```python
from build123d import *

# Parameters (mm, degrees)
ZAOBLIT1_R = 20


with BuildPart() as part:
    # Skica1 → Rotovat1 (revolve)
    with BuildSketch(Plane.XY, mode=Mode.PRIVATE) as rotovat1_sk:
        Polygon((0, 0), (0, 44.5), (349.599506462, 44.5), (372.134762873, 17.400641026), (420, 17.400641026), (420, 0), align=None)
    revolve(rotovat1_sk.sketch.rotate(Axis((0, 0, 0), (1, 0, 0)), 90), axis=Axis((0, 0, 0), (1, 0, 0)))

    # Zaoblit1
    zaoblit1_edges = [part.edges().sort_by_distance(p)[0] for p in [
        (372.134762873, 0, -17.400641026),
        (349.599506462, 0, -44.5),
        (0, 0, -44.5),
    ]]
    fillet(zaoblit1_edges, radius=ZAOBLIT1_R)


solid = part.part
```
Geometry check sheet. Reference: the model listing, model coordinates, mm. A direction names the side the tool comes from. Give positions to 0.01 mm unless a question says otherwise; leave off trailing zeros. Loops run counter-clockwise (first coordinate to the right, second up) from the corner with the lowest first, then second, coordinate; pieces in that order, holes last. Notation, with made-up numbers: M 42.5,74.5 L 62.5,74.5 A19 ccw 62.5,90.5 Z; hole C 25.25,87 d1. An arc over 180 degrees is marked long. Answer as CSV lines item,"result".
Item 1: Material ranges on line 1 (Y direction, x = 397, z = -2); line 2 (X direction, y = 1, z = -31.5); line 3 (Y direction, x = 102, z = 11), recorded low to high.
Values:
line 1,"y = -17.29 to 17.29"
line 2,"x = 1.27 to 360.4"
line 3,"y = -43.12 to 43.12"
Item 2: Depth check by flat-ended pin: P1, Ø6, axis at x = 118, z = 10.5, coming from the +Y side; P2, Ø5, axis at x = 236.5, z = -29, coming from the +Y side; P3, Ø1.5, axis at y = 23, z = -3, coming from the +X side. Enter the tip coordinate at first touch or a pass-through.
Values:
P1,"stops at y = 43.86"
P2,"stops at y = 35.75"
P3,"stops at x = 368.24"
Item 3: Access from +Z, -Z, +X, -X, +Y, -Y to the whole of each face (thin tool, end or side, straight path). Record for faces 1 (the cylindrical face through (401.027, 16.987, -3.772)), 2 (the flat face through (420, 0, 0)).
Values:
face 1,"+X"
face 2,"+Z, -Z, +X, +Y, -Y"
Item 4: Cross-section at A-A on x = 291. Record the cut outline in (y, z).
Values:
outline,"C 0,0 d89"
